from build123d import *

# Parameters (mm, degrees)
BOSS_EXTRU_1_DEPTH      = 5
ESQUISSE2_R             = 5.1
ESQUISSE2_R_2           = 2.1
ENL_V_MAT_EXTRU_1_DEPTH = 81.777472107
ESQUISSE3_W             = 24
ESQUISSE3_H             = 20
BOSS_EXTRU_2_DEPTH      = 20
CHANFREIN1_SIZE         = 10
ESQUISSE4_W             = 36
ESQUISSE4_H             = 10
ENL_V_MAT_EXTRU_2_DEPTH = 20
ESQUISSE5_R             = 2.1
ENL_V_MAT_EXTRU_3_DEPTH = 87.168439698
CONG_1_R                = 8
ESQUISSE6_R             = 5.5
ENL_V_MAT_EXTRU_4_DEPTH = 2
CHANFREIN2_SIZE         = 1
CONG_4_R                = 2


with BuildPart() as part:
    # Esquisse1 → Boss.-Extru.1 (new body)
    with BuildSketch(Plane.XY):
        with BuildLine():
            Line((-70, 10), (70, 10))
            ThreePointArc((70, 10), (80, 0), (70, -10))
            Line((70, -10), (-70, -10))
            ThreePointArc((-70, -10), (-80, 0), (-70, 10))
        make_face()
    extrude(amount=BOSS_EXTRU_1_DEPTH)

    # Esquisse2 → Enlèv. mat.-Extru.1 (cut, through all)
    with BuildSketch(Plane.XY.offset(5)):
        with Locations((-70, 0)):
            Circle(ESQUISSE2_R)
        with Locations((70, 0)):
            Circle(ESQUISSE2_R)
        with Locations((-50, 0)):
            Circle(ESQUISSE2_R_2)
        with Locations((50, 0)):
            Circle(ESQUISSE2_R_2)
    extrude(amount=-ENL_V_MAT_EXTRU_1_DEPTH, mode=Mode.SUBTRACT)

    # Esquisse3 → Boss.-Extru.2 (add)
    with BuildSketch(Plane.XY.offset(5)):
        Rectangle(ESQUISSE3_W, ESQUISSE3_H)
    extrude(amount=BOSS_EXTRU_2_DEPTH)

    # Chanfrein1
    chanfrein1_edges = [part.edges().sort_by_distance(p)[0] for p in [
        (12, 0, 5),
        (-12, 0, 5),
    ]]
    chamfer(chanfrein1_edges, length=CHANFREIN1_SIZE)

    # Esquisse4 → Enlèv. mat.-Extru.2 (cut)
    with BuildSketch(Plane.XY.offset(25)):
        Rectangle(ESQUISSE4_W, ESQUISSE4_H)
    extrude(amount=-ENL_V_MAT_EXTRU_2_DEPTH, mode=Mode.SUBTRACT)

    # Esquisse5 → Enlèv. mat.-Extru.3 (cut, through all)
    with BuildSketch(Plane(origin=(0, 10, 0), x_dir=(1, 0, 0), z_dir=(0, 1, 0))):
        with Locations(Location((0, -17, 0), (0, 0, 270))):
            Circle(ESQUISSE5_R)
    extrude(amount=-ENL_V_MAT_EXTRU_3_DEPTH, mode=Mode.SUBTRACT)

    # Congé1
    cong_1_edges = [part.edges().sort_by_distance(p)[0] for p in [
        (-22, 0, 5),
        (-12, -7.5, 25),
        (12, -7.5, 25),
        (22, 0, 5),
        (-12, 7.5, 25),
        (12, 7.5, 25),
    ]]
    fillet(cong_1_edges, radius=CONG_1_R)

    # Esquisse6 → Enlèv. mat.-Extru.4 (cut)
    with BuildSketch(Plane(origin=(0, 10, 0), x_dir=(1, 0, 0), z_dir=(0, 1, 0))):
        with Locations(Location((0, -17, 0), (0, 0, 270))):
            Circle(ESQUISSE6_R)
    extrude(amount=-ENL_V_MAT_EXTRU_4_DEPTH, mode=Mode.SUBTRACT)

    # Chanfrein2
    chanfrein2_edges = [part.edges().sort_by_distance(p)[0] for p in [
        (0, 10, 11.5),
    ]]
    chamfer(chanfrein2_edges, length=CHANFREIN2_SIZE)

    # Congé4
    # the kernel refuses this fillet: 2 mm, written as the material it takes off along each edge
    with BuildSketch(Plane(origin=(18, -5, 9), x_dir=(0.7394878589424565, 0, -0.6731698942144558), z_dir=(0, 1, 0)), Plane(origin=(-18, 5, 9), x_dir=(-0.7394878589424565, 0, -0.6731698942144557), z_dir=(0, -1, 0))) as cong_4_piece_1:
        with BuildLine():
            CenterArc((4.431818389, 1.970329953), CONG_4_R, 150.40864019, 109.709922664)
            Line((2.692679577, 2.957951436), (2.518765696, 3.056713584))
            ThreePointArc((2.518765696, 3.056713584), (1.198442217, 1.613609697), (-0.147897572, 0.134633979))
            Line((-0.147897572, 0.134633979), (0.009378777, -0.199779975))
            ThreePointArc((0.009378777, -0.199779975), (2.349946778, -0.089900774), (4.054276537, -0.197032995))
            Line((4.054276537, -0.197032995), (4.088598523, 0))
        make_face()
    extrude(amount=10, mode=Mode.SUBTRACT)


solid = part.part
Work out the finished part from the listing and answer in its coordinate system (mm). A direction names the side the tool comes from. Coordinates: 2 decimals unless noted, no trailing zeros. Write each loop counter-clockwise with the first axis right and the second up, starting at its lowest first coordinate (ties: lowest second). Pieces come first, ordered by that corner, then holes. Notation, with made-up numbers: (69, 61.5) - (108, 61.5) arc R14 ccw to (108, 87.5) - close; hole circle Ø2 at (41, 78.5). An arc over 180 degrees is marked (long way). One line per question, with ' | ' between items.
1) Find section D-D, the plane x = -66.5. Determine the outline of the cut face in (y, z).
Checks:
outline: (-10, 0) - (-3.71, 0) - (-3.71, 5) - (-10, 5) - close; (3.71, 0) - (10, 0) - (10, 5) - (3.71, 5) - close
2) The mould has two halves that part along X. Classify faces 4 (the face through (22.293, 0.14, 5.592)), 5 (the face through (0, 0, 5)), 6 (the face through (53, 0, 5)): +X half, -X half, draft (parallel to the pull), parting line (faces both ways), or undercut.
Checks:
face 4: +X half | face 5: undercut | face 6: draft
3) Find section C-C, the plane x = 50. Determine the outline of the cut face in (y, z), and give its area (3 significant figures).
Checks:
outline: (-10, 0) - (-2.1, 0) - (-2.1, 5) - (-10, 5) - close; (2.1, 0) - (10, 0) - (10, 5) - (2.1, 5) - close | area: 79.0 mm2
4) Find section A-A, the plane x = 0. Determine the outline of the cut face in (y, z).
Checks:
outline: (-10, 0) - (10, 0) - (10, 10.5) - (9, 11.5) - (8, 11.5) - (8, 14.9) - (5, 14.9) - (5, 5) - (-5, 5) - (-5, 14.9) - (-10, 14.9) - close; (-10, 19.1) - (-5, 19.1) - (-5, 25) - (-10, 25) - close; (5, 19.1) - (8, 19.1) - (8, 22.5) - (9, 22.5) - (10, 23.5) - (10, 25) - (5, 25) - close
5) Consider probe 1 along Y at (x, z) = (13, 8); probe 2 along X at (y, z) = (7.75, 17.25); probe 3 along Y at (x, z) = (70, 1.2). Determine where each line is inside the solid, lowest interval first. Write a range as [from, to].
Checks:
probe 1: [-10, -5], [5, 10] | probe 2: [-12, -2.09], [2.09, 12] | probe 3: [-10, -5.1], [5.1, 10]
6) Flat-ended cylindrical pins translate along their axes: P1, Ø6, axis at x = 48, y = 0.5, coming from the +Z side; P2, Ø5, axis at y = 4.5, z = 6, coming from the -X side; P3, Ø0.6, axis at y = -8.5, z = 16, coming from the -X side. Find the tip coordinate at first contact, or state that the pin passes through.
Checks:
P1: z = 5 | P2: x = -79.75 | P3: x = -12
7) Find section B-B, the plane y = -3.5. Determine the outline of the cut face in (x, z), and give its area (3 significant figures).
Checks:
outline: (-79.37, 0) - (-73.71, 0) - (-73.71, 5) - (-79.37, 5) - close; (-66.29, 0) - (66.29, 0) - (66.29, 5) - (25.31, 5) arc R8 cw to (21.02, 6.25) arc R2 ccw to (18, 5) - (-18, 5) arc R2 ccw to (-21.02, 6.25) arc R8 cw to (-25.31, 5) - (-66.29, 5) - close; (73.71, 0) - (79.37, 0) - (79.37, 5) - (73.71, 5) - close | area: 731 mm2
8) For faces 1 (the face through (0, -5, 14)), 2 (the face through (1, 0, 0)), 3 (the face through (-4.9, 8.5, 19.5)), determine the directions among +Z, -Z, +X, -X, +Y, -Y from which every point of the face is accessible in a straight line to the end or side of a thin tool.
Checks:
face 1: +Z | face 2: -Z, +X, -X, +Y, -Y | face 3: +Y
